from build123d import *

# Parameters (mm, degrees)
BOSS_EXTRUDE1_DEPTH      = 5
BOSS_EXTRUDE1_DEPTH_BACK = 5
SKETCH1_W                = 10
SKETCH1_H                = 10
SKETCH2_R                = 4.1
CUT_EXTRUDE1_DEPTH       = 2
SKETCH5_R                = 4.1
CUT_EXTRUDE2_DEPTH       = 2
SKETCH6_R                = 4.1
CUT_EXTRUDE3_DEPTH       = 2


with BuildPart() as part:
    # Sketch1 → Boss-Extrude1 (new, two sides: drawn at the far end of the back side and taken through both)
    with BuildSketch(Plane.XY.offset(-BOSS_EXTRUDE1_DEPTH_BACK)):
        Rectangle(SKETCH1_W, SKETCH1_H)
    extrude(amount=BOSS_EXTRUDE1_DEPTH + BOSS_EXTRUDE1_DEPTH_BACK)

    # Sketch2 → Cut-Extrude1 (cut)
    with BuildSketch(Plane(origin=(0, 5, 0), x_dir=(1, 0, 0), z_dir=(0, 1, 0))):
        with Locations(Location((0, 0, 0), (0, 0, 180))):
            Circle(SKETCH2_R)
    extrude(amount=-CUT_EXTRUDE1_DEPTH, mode=Mode.SUBTRACT)

    # Sketch5 → Cut-Extrude2 (cut)
    with BuildSketch(Plane.XY.offset(5)):
        Circle(SKETCH5_R)
    extrude(amount=-CUT_EXTRUDE2_DEPTH, mode=Mode.SUBTRACT)

    # Sketch6 → Cut-Extrude3 (cut)
    with BuildSketch(Plane(origin=(5, 0, 0), x_dir=(0, 0, -1), z_dir=(1, 0, 0))):
        Circle(SKETCH6_R)
    extrude(amount=-CUT_EXTRUDE3_DEPTH, mode=Mode.SUBTRACT)


solid = part.part
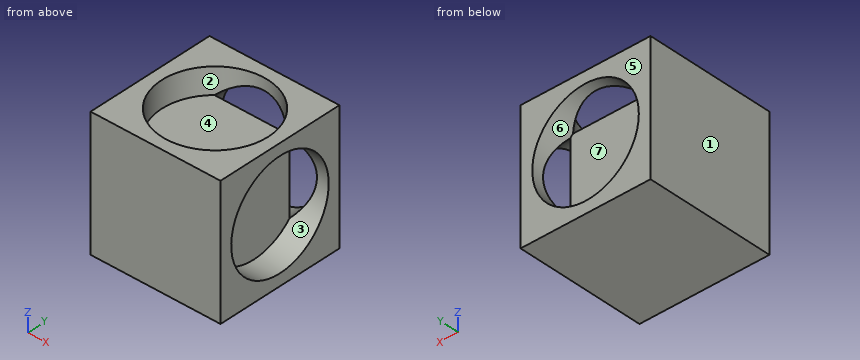
Design review of the part built by this model. Coordinates are the model's own, in mm. Face numbers are marked on the shaded views. A direction names the side the tool comes from. Round coordinates to 2 decimals unless told otherwise and drop trailing zeros. Write each loop counter-clockwise with the first axis right and the second up, starting at its lowest first coordinate (ties: lowest second). Pieces come first, ordered by that corner, then holes. Notation, with made-up numbers: (-15.5, 12) -> (16.5, 12) arc R11 ccw to (16.5, 18) -> close; hole circle Ø2 at (23, -34). An arc over 180 degrees is marked (long way). One line per item, written item: value. Start each with the question number.
Q1. Insertion check: P1, Ø2, axis at y = 0, z = 1, coming from the +X side; P2, Ø2, axis at x = -1.5, y = 0, coming from the +Z side; P3, Ø5.5, axis at x = 0.5, z = -1, coming from the +Y side. Each pin has a flat end and moves straight along its axis. Give the tip position at first contact, or say it passes through.
Q2. Add section C-C (z = 4.25). Give the boundary of the cut face in (x, y), then the cut area to 3 significant figures.
Q3. Tool access review of the marked faces 1, 2 and 3: name each direction out of +Z, -Z, +X, -X, +Y, -Y from which nothing blocks a thin tool from reaching the whole face with its end or side.
Q4. The part is to be moulded in two halves that separate along Z. For the marked faces 4, 5, 6 and 7, say which applies: pulls with the +Z half, pulls with the -Z half, needs draft (parallel to the pull), parting line crosses it, or undercut.
Q5. Add section A-A (x = 0). Give the boundary of the cut face in (y, z), then the cut area to 3 significant figures.
Q6. To check wall thickness, follow probe 1 along Y at (x, z) = (4.2, 0); probe 2 along X at (y, z) = (0.25, 1). State the ranges of each line that lie inside material, in increasing order.
Response:
1. P1: stops at x = 3
1. P2: stops at z = 3
1. P3: stops at y = 3
2. outline: (-5, -5) -> (5, -5) -> (5, 5) -> (-5, 5) -> close; hole circle Ø8.2 at (0, 0)
2. area: 47.2 mm^2
3. face 1: +Z, -Z, -X, +Y, -Y
3. face 2: +Z
3. face 3: +X
4. face 4: pulls with the +Z half
4. face 5: needs draft
4. face 6: undercut
4. face 7: undercut
5. outline: (-5, -5) -> (5, -5) -> (5, -4.1) -> (3, -4.1) -> (3, 3) -> (-4.1, 3) -> (-4.1, 5) -> (-5, 5) -> close; (4.1, 4.1) -> (5, 4.1) -> (5, 5) -> (4.1, 5) -> close
5. area: 68.4 mm^2
6. probe 1: y = -5 to -4.1, 4.1 to 5
6. probe 2: x = -5 to 3
